from build123d import *
from OCP.BRepFilletAPI import BRepFilletAPI_MakeChamfer

# Parameters (mm, degrees)
DIAM_TRE_DU_PER_AGE_3_0_3_1_D     = 3
DIAM_TRE_DU_PER_AGE_3_0_3_1_DEPTH = 32.45
CHANFREIN1_SIZE                   = 0.5
CHANFREIN2_SIZE                   = 0.2
CHANFREIN3_SIZE                   = 0.173205081
CHANFREIN3_SIZE2                  = 0.3
CHANFREIN4_SIZE                   = 0.3
CHANFREIN4_SIZE2                  = 0.173205081
CONG_1_R                          = 0.2
ESQUISSE6_W                       = 8
ESQUISSE6_H                       = 1.5
ENL_V_MAT_EXTRU_1_DEPTH           = 12


with BuildPart() as part:
    # Esquisse1 → Révolution1 (revolve)
    with BuildSketch(Plane.XY, mode=Mode.PRIVATE) as r_volution1_sk:
        Polygon((-3, 10.4), (-3, 0), (29.45, 0), (29.45, 3), (12.8, 3), (12.8, 2.85), (12, 2.85), (12, 3), (0.996794919, 3), (0.623589838, 2.9), (0, 2.9), (0, 10.4), align=None)
    revolve(r_volution1_sk.sketch.rotate(Axis((-3, 0, 0), (1, 0, 0)), 270), axis=Axis((-3, 0, 0), (1, 0, 0)))

    # Diamètre du perçage Ø3.0 (3)1
    with Locations(Plane.ZY.offset(3)):
        with Locations((-6.819950055, -3.9375), (6.819950055, -3.9375), (0, 7.875)):
            Hole(DIAM_TRE_DU_PER_AGE_3_0_3_1_D / 2, depth=DIAM_TRE_DU_PER_AGE_3_0_3_1_DEPTH)

    # Esquisse4 → Perçage1 (revolve, cut)
    with BuildSketch(Plane(origin=(-3, 0, 0), x_dir=(0, 0, 1), z_dir=(0, 1, 0))):
        Polygon((0, 0), (0, 0.5), (4.866025404, 0.5), (5, 0), align=None)
    revolve(axis=Axis((107, 0, 0), (-1, 0, 0)), mode=Mode.SUBTRACT)

    # Chanfrein1
    chanfrein1_edges = [part.edges().sort_by_distance(p)[0] for p in [
        (29.45, 0, 3),
    ]]
    chamfer(chanfrein1_edges, length=CHANFREIN1_SIZE)

    # Chanfrein2
    chanfrein2_edges = [part.edges().sort_by_distance(p)[0] for p in [
        (-3, 0, 10.4),
        (0, 0, 10.4),
    ]]
    chamfer(chanfrein2_edges, length=CHANFREIN2_SIZE)

    # Chanfrein3
    chanfrein3_edges = [part.edges().sort_by_distance(p)[0] for p in [
        (-3, 7.875, 1.5),
    ]]
    chanfrein3_side = [part.faces().sort_by_distance(p)[0] for p in [
        (-3, 0, 9.911500433),
    ]]
    chamfer(chanfrein3_edges, length=CHANFREIN3_SIZE, length2=CHANFREIN3_SIZE2, reference=chanfrein3_side[0])

    # Chanfrein4: one chamfer whose edges measure the first distance from different faces: ONE call of the kernel's chamfer builder (chamfer() names one face for all edges)
    chanfrein4_edges_1 = [part.edges().sort_by_distance(p)[0] for p in [
        (-3, -3.9375, 8.319950055),
    ]]
    chanfrein4_side_1 = [part.faces().sort_by_distance(p)[0] for p in [
        (-1.5, -3.9375, 8.319950055),
    ]]
    chanfrein4_edges_2 = [part.edges().sort_by_distance(p)[0] for p in [
        (-3, -3.9375, -5.319950055),
    ]]
    chanfrein4_side_2 = [part.faces().sort_by_distance(p)[0] for p in [
        (-1.5, -3.9375, -5.319950055),
    ]]
    chanfrein4 = BRepFilletAPI_MakeChamfer(part.part.solid().wrapped)
    for e in chanfrein4_edges_1:
        chanfrein4.Add(CHANFREIN4_SIZE, CHANFREIN4_SIZE2, e.wrapped, chanfrein4_side_1[0].wrapped)  # the first distance lies on this face
    for e in chanfrein4_edges_2:
        chanfrein4.Add(CHANFREIN4_SIZE, CHANFREIN4_SIZE2, e.wrapped, chanfrein4_side_2[0].wrapped)  # the first distance lies on this face
    add(Compound.cast(chanfrein4.Shape()), mode=Mode.REPLACE)

    # Congé1
    cong_1_edges = [part.edges().sort_by_distance(p)[0] for p in [
        (0, 0, 2.9),
        (0.623589838, 0, 2.9),
    ]]
    fillet(cong_1_edges, radius=CONG_1_R)

    # Esquisse6 → Enlèv. mat.-Extru.1 (cut)
    with BuildSketch(Plane(origin=(29.45, 0, 0), x_dir=(0, 0, -1), z_dir=(1, 0, 0))):
        with Locations((0, 3.25)):
            Rectangle(ESQUISSE6_W, ESQUISSE6_H)
    extrude(amount=-ENL_V_MAT_EXTRU_1_DEPTH, mode=Mode.SUBTRACT)


solid = part.part
Build history of the part. All positions in model axes, mm. A direction names the side the tool comes from. Give positions to 0.01 mm unless a question says otherwise; leave off trailing zeros. Order: outer loops, then holes, each group sorted by start corner. A loop starts at its lowest first (then second) coordinate and runs counter-clockwise, first axis right, second up. Notation, with made-up numbers: M 45,-14.5 L 86,-14.5 A15 ccw 86,13.5 Z; hole C -27.75,86.5 d9. An arc over 180 degrees is marked long. Use one line per item in the form item = value.
Q1. Wall check: probe 1 along X at (y, z) = (6, 4.25); probe 2 along X at (y, z) = (-3, 1.5); probe 3 along Z at (x, y) = (19.5, 1). Give the ranges that are in metal, low to high.
Conclusion:
probe_1 = -3 to 0
probe_2 = -2.5 to 0
probe_3 = -2.83 to 2.83
Q2. Slice it at A-A, the plane x = 9. Write the cut outline in (y, z).
Conclusion:
outline = C 0,0 d6
Q3. Pull direction Y, two halves, no side cores. Call faces 1 (the cylindrical face through (20.76, -2.93, 0.65)), 2 (the flat face through (0, 2.4, -2.4)), 3 (the cylindrical face through (-1.33, 6.41, 0.33)): released by +Y, released by -Y, zero draft, split by the parting line, or undercut.
Conclusion:
face_1 = split by the parting line
face_2 = zero draft
face_3 = undercut
Q4. Pin check, flat tips, straight feed: P1, Ø6.5, axis at y = 1.5, z = 0, coming from the -X side; P2, Ø10.5, axis at y = 1, z = 2, coming from the -X side; P3, Ø2.5, axis at y = -3.94, z = 6.82, coming from the -X side; P4, Ø1, axis at x = 9.5, y = -1.5, coming from the +Z side. Stop position of each tip, or through.
Conclusion:
P1 = -2.5
P2 = -3
P3 = through
P4 = 2.83
Q5. Which spindle directions (+Z, -Z, +X, -X, +Y, -Y) get a long thin tool onto all of the face, cutting with end or side? Do faces 4 (the flat face through (-2.5, 0, 0)), 5 (the cylindrical face through (0.396, 2.445, -1.559)), 6 (the cylindrical face through (6.42, 0.9, -2.86)). Say none if no direction does.
Conclusion:
face_4 = -X
face_5 = none
face_6 = +X
